The drawing under review shows one solid part. Ordinate dimensions are in mm from its lowest x, y, z. Give positions to 0.01 mm unless a question says otherwise; leave off trailing zeros. Order: outer loops, then holes, each group sorted by start corner. A loop starts at its lowest first (then second) coordinate and runs counter-clockwise, first axis right, second up. Notation, with made-up numbers: (31.5, 67.5) -> (81.5, 67.5) arc R10 ccw to (81.5, 72.5) -> close; hole circle Ø7 at (45.25, 89.25). An arc over 180 degrees is marked (long way). Return JSON: item names as keys, results as strings. Group by question number.
1) The part is to be moulded in two halves that separate along Y. For the marked faces 1 and 2, say which applies: released by +Y, released by -Y, zero draft, split by the parting line, or undercut.
2) Insertion check: P1, Ø0.6, axis at x = 2.5, y = 4.5, coming from the +Z side; P2, Ø0.9, axis at x = 3, z = 27.5, coming from the +Y side. Each pin has a flat end and moves straight along its axis. Give the tip position at first contact, or say it passes through.
3) Add section B-B (z = 28). Give the boundary of the cut face in (x, y).
4) Add section A-A (x = 2.5). Give the boundary of the cut face in (y, z), then the cut area to 3 significant figures.
5) To check wall thickness, follow line 1 along X through (y, z) = (4, 21); line 2 along X through (y, z) = (2.35, 18); line 3 along Z through (x, y) = (4.25, 1.25). State the ranges of each line that lie inside material, in increasing order.
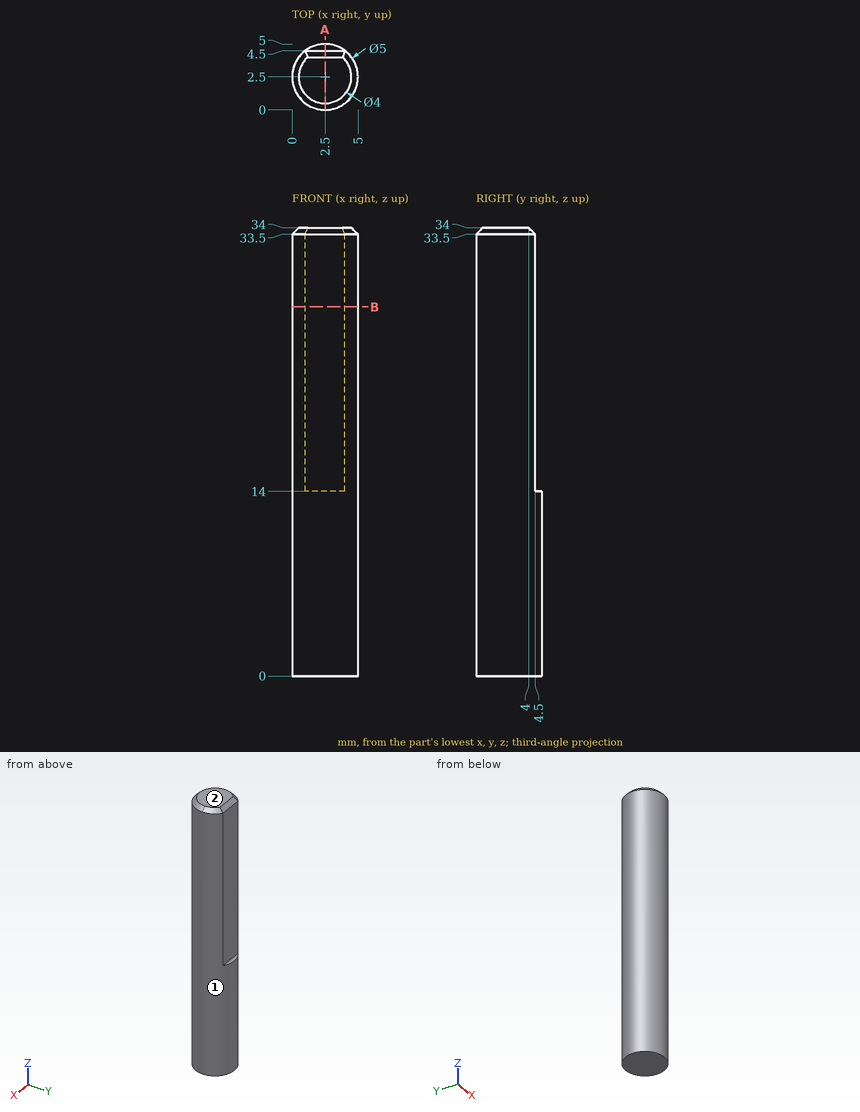
Evaluation:
{
 "1": {"face 1": "split by the parting line", "face 2": "zero draft"},
 "2": {"P1": "z = 33.8", "P2": "y = 4.5"},
 "3": {"outline": "(1, 4.5) arc R2.5 ccw (long way) to (4, 4.5) -> close"},
 "4": {"outline": "(0, 0) -> (5, 0) -> (5, 14) -> (4.5, 14) -> (4.5, 33.5) -> (4, 34) -> (0.5, 34) -> (0, 33.5) -> close", "area": "160 mm^2"},
 "5": {"line 1": "0.5 to 4.5", "line 2": "0 to 5", "line 3": "0 to 33.85"}
}
